The model under review builds one solid part; all positions refer to its coordinate system, in mm. A direction names the side the tool comes from. Coordinates: 2 decimals unless noted, no trailing zeros. Order: outer loops, then holes, each group sorted by start corner. A loop starts at its lowest first (then second) coordinate and runs counter-clockwise, first axis right, second up. Notation, with made-up numbers: M 19,71 L 59,71 A18 ccw 59,101 Z; hole C 35.5,17 d11. An arc over 180 degrees is marked long. Write each question's results on one line, items separated by ' | '.
Autodesk Inventor part; units mm, degrees
ref_plane "YZ Plane" through (0, 0, 0) normal (1, 0, 0) x (0, 1, 0)
ref_plane "XZ Plane" through (0, 0, 0) normal (0, 1, 0) x (-1, 0, 0)
ref_plane "XY Plane" through (0, 0, 0) normal (0, 0, 1) x (1, 0, 0)
sketch "Sketch1" plane through (0, 0, 0) normal (0, 0, 1) x (1, 0, 0)
  line L0 (0, 0) -> (43, 0)
  line L1 (43, 0) -> (43, 20)
  line L2 (43, 20) -> (0, 20)
  line L3 (0, 20) -> (0, 0)
  dimension "d0" = 43
  dimension "d1" = 20
extrude "Extrusion1" add sketch "Sketch1" along normal blind 2
sketch "Sketch2" plane through (0, 0, 0) normal (0, -1, 0) x (1, 0, 0)
  line L0 (43, 0) -> (43, 2)
  line L1 (0, 0) -> (0, 2)
  line L2 (0, 0) -> (-2, 0)
  line L3 (-2, 0) -> (0, 2)
  line L4 (43, 0) -> (45, 0)
  line L5 (45, 0) -> (43, 2)
  dimension "d4" = 2
  dimension "d5" = 2
extrude "Extrusion2" add sketch "Sketch2" against normal blind 20
sketch "Sketch3" plane through (0, 0, 2) normal (0, 0, 1) x (1, 0, 0)
  line L0 (0, 0) -> (43, 0)
  line L1 (43, 0) -> (43, 20)
  line L2 (43, 20) -> (0, 20)
  line L3 (0, 20) -> (0, 0)
  line L4 (9, 3.5) -> (34, 3.5)
  line L5 (34, 3.5) -> (34, 16.5)
  line L6 (34, 16.5) -> (9, 16.5)
  line L7 (9, 16.5) -> (9, 3.5)
  dimension "d8" = 25
  dimension "d9" = 13
  dimension "d10" = 3.5
  dimension "d11" = 3.5
  dimension "d12" = 9
  dimension "d13" = 9
extrude "Extrusion3" cut sketch "Sketch3" against normal blind 1.5 contours L7 L6 L5 L4
sketch "Sketch4" plane through (0, 0, 2) normal (0, 0, 1) x (1, 0, 0)
  line L0 (34, 16.5) -> (34, 3.5)
  line L1 (34, 3.5) -> (15, 3.5)
  line L2 (15, 3.5) -> (15, 8)
  line L3 (15, 8) -> (34, 8)
  line L4 (34, 8) -> (34, 3.5)
  line L5 (9, 16.5) -> (34, 16.5)
  line L6 (34, 16.5) -> (15, 16.5)
  line L7 (15, 16.5) -> (15, 12)
  line L8 (15, 12) -> (34, 12)
  line L9 (34, 12) -> (34, 16.5)
  dimension "d16" = 19
  dimension "d17" = 4.5
  dimension "d18" = 4.5
extrude "Extrusion4" add sketch "Sketch4" against normal blind 1.49
chamfer "Chamfer5" distance 4.5 distance2 1.49 1 edges at (24.5, 12, 0.51) measured on face at (21.3333, 15, 0.51)
chamfer "Chamfer6" distance 4.5 distance2 1.49 1 edges at (24.5, 8, 0.51) measured on face at (27.6667, 5, 0.51)
properties part number "deksel token Nieuw bevestiging"
1) Take a section at C-C on z = 1.5. State the section outline as (x, y) points.
Solutions:
outline: M -0.5,0 L 43.5,0 L 43.5,20 L -0.5,20 Z; hole M 9,3.5 L 15,3.5 L 15,6.49 L 34,6.49 L 34,13.51 L 15,13.51 L 15,16.5 L 9,16.5 Z
2) For faces 4 (the flat face through (15, 5.2, 1.4)), 5 (the flat face through (21, 10, 0)), 6 (the flat face through (34, 10, 1)), list the 3-axis set-ups (+Z, -Z, +X, -X, +Y, -Y) from which the entire face can be reached by the end or side of a thin tool; tool diameter is ignored.
Solutions:
face 4: +Z | face 5: -Z, +X, -X, +Y, -Y | face 6: none
3) The part is to be moulded in two halves that separate along Y. For faces 1 (the flat face through (11, 16.5, 1)), 2 (the flat face through (22, 20, 1)), 3 (the flat face through (44, 10, 1)), say which applies: pulls with the +Y half, pulls with the -Y half, needs draft (parallel to the pull), parting line crosses it, or undercut.
Solutions:
face 1: undercut | face 2: pulls with the +Y half | face 3: needs draft
4) Take a section at D-D on y = 7.5. State the section outline as (x, z) points.
Solutions:
outline: M -2,0 L 45,0 L 43,2 L 15,2 L 15,1.83 L 34,1.83 L 34,0.5 L 9,0.5 L 9,2 L 0,2 Z
5) For pin 1 (0.8 mm diameter, centred on y = 7, z = 1, fed in from -X); pin 2 (1.2 mm diameter, centred on y = 15.5, z = 1.5, fed in from -X), all flat-tipped, find the tip position at first contact; note any pin that passes through.
Solutions:
pin 1: x = -1.4 | pin 2: x = -1.1
6) To check wall thickness, follow line 1 along Y through (x, z) = (14, 1.6); line 2 along X through (y, z) = (16, 1.45); line 3 along X through (y, z) = (7.75, 1.1). State the ranges of each line that lie inside material, in increasing order.
Solutions:
line 1: 0 to 3.5, 16.5 to 20 | line 2: -0.55 to 9, 15 to 43.55 | line 3: -0.9 to 9, 34 to 43.9
7) Take a section at B-B on y = 15.5. State the section outline as (x, z) points.
Solutions:
outline: M -2,0 L 45,0 L 43,2 L 15,2 L 15,0.84 L 34,0.84 L 34,0.5 L 9,0.5 L 9,2 L 0,2 Z
